Part model, mm, in its own coordinate system. Give positions to 0.01 mm unless a question says otherwise; leave off trailing zeros. Order: outer loops, then holes, each group sorted by start corner. A loop starts at its lowest first (then second) coordinate and runs counter-clockwise, first axis right, second up. Notation, with made-up numbers: M -16,68.5 L 19,68.5 A19 cw 19,99.5 Z; hole C -22,74.5 d8. An arc over 180 degrees is marked long. One line per question, with ' | ' between items.
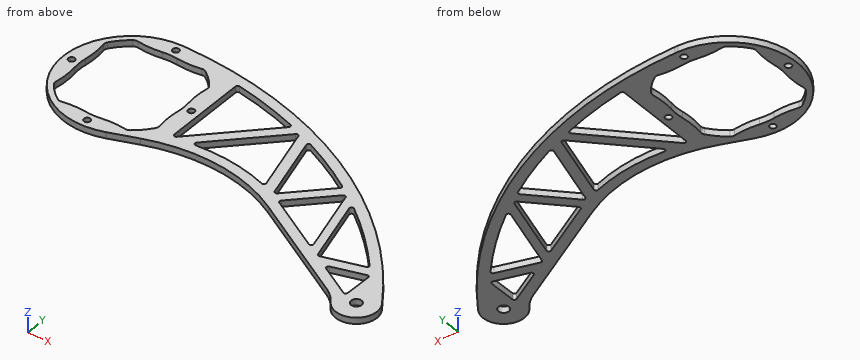
```python
from build123d import *

# Parameters (mm, degrees)
SKETCH_2_R          = 1.55
EXTRUDE_1_DEPTH     = 3
SKETCH_7_R          = 2.55
CUT_EXTRUDE_2_DEPTH = 5
CUT_EXTRUDE_4_DEPTH = 184.170177924
CUT_EXTRUDE_5_DEPTH = 184.170177924


with BuildPart() as part:
    # 草图2 → 凸台-拉伸1 (new body)
    with BuildSketch(Plane.XY):
        with BuildLine():
            Line((10.730362356, -31.206719208), (23.987000349, -26.648453139))
            ThreePointArc((23.987000349, -26.648453139), (58.3964084, -22.742948884), (91.232460283, -33.745404185))
            Line((91.232460283, -33.745404185), (142.367635598, -64.500382059))
            ThreePointArc((142.367635598, -64.500382059), (145.885654628, -67.188078585), (148.726187194, -70.583891486))
            ThreePointArc((148.726187194, -70.583891486), (162.505343691, -73.443257489), (165.49953058, -59.692767585))
            ThreePointArc((165.49953058, -59.692767585), (95.05641772, 7.182197604), (1.414573065, 32.983322541))
            ThreePointArc((1.414573065, 32.983322541), (0.707335687, 32.99583049), (0, 33))
            ThreePointArc((0, 33), (-32.548592395, -5.439589421), (10.730362356, -31.206719208))
        make_face()
        with Locations((-29, 0)):
            Circle(SKETCH_2_R, mode=Mode.SUBTRACT)
        with Locations((0, 29)):
            Circle(SKETCH_2_R, mode=Mode.SUBTRACT)
        with Locations((0, -29)):
            Circle(SKETCH_2_R, mode=Mode.SUBTRACT)
        with Locations((29, 0)):
            Circle(SKETCH_2_R, mode=Mode.SUBTRACT)
        with BuildLine():
            ThreePointArc((-17.479158967, 24.504877103), (-21.283914114, 21.283914114), (-24.504877103, 17.479158967))
            ThreePointArc((-24.504877103, 17.479158967), (-24.920981627, 16.556612715), (-24.953330783, 15.545085111))
            ThreePointArc((-24.953330783, 15.545085111), (-24.421536801, 9.520350069), (-24.806472783, 3.484452336))
            ThreePointArc((-24.806472783, 3.484452336), (-25.05, 0), (-24.806472783, -3.484452336))
            ThreePointArc((-24.806472783, -3.484452336), (-24.421536801, -9.520350069), (-24.953330783, -15.545085111))
            ThreePointArc((-24.953330783, -15.545085111), (-24.920981627, -16.556612715), (-24.504877103, -17.479158967))
            ThreePointArc((-24.504877103, -17.479158967), (-21.283914114, -21.283914114), (-17.479158967, -24.504877103))
            ThreePointArc((-17.479158967, -24.504877103), (-16.556612715, -24.920981627), (-15.545085111, -24.953330783))
            ThreePointArc((-15.545085111, -24.953330783), (-9.520350069, -24.421536801), (-3.484452336, -24.806472783))
            ThreePointArc((-3.484452336, -24.806472783), (0, -25.05), (3.484452336, -24.806472783))
            ThreePointArc((3.484452336, -24.806472783), (9.520350069, -24.421536801), (15.545085111, -24.953330783))
            ThreePointArc((15.545085111, -24.953330783), (16.556612715, -24.920981627), (17.479158967, -24.504877103))
            ThreePointArc((17.479158967, -24.504877103), (21.283914114, -21.283914114), (24.504877103, -17.479158967))
            ThreePointArc((24.504877103, -17.479158967), (24.920981627, -16.556612715), (24.953330783, -15.545085111))
            ThreePointArc((24.953330783, -15.545085111), (24.421536801, -9.520350069), (24.806472783, -3.484452336))
            ThreePointArc((24.806472783, -3.484452336), (25.05, 0), (24.806472783, 3.484452336))
            ThreePointArc((24.806472783, 3.484452336), (24.421536801, 9.520350069), (24.953330783, 15.545085111))
            ThreePointArc((24.953330783, 15.545085111), (24.920981627, 16.556612715), (24.504877103, 17.479158967))
            ThreePointArc((24.504877103, 17.479158967), (21.283914114, 21.283914114), (17.479158967, 24.504877103))
            ThreePointArc((17.479158967, 24.504877103), (16.556612715, 24.920981627), (15.545085111, 24.953330783))
            ThreePointArc((15.545085111, 24.953330783), (9.520350069, 24.421536801), (3.484452336, 24.806472783))
            ThreePointArc((3.484452336, 24.806472783), (0, 25.05), (-3.484452336, 24.806472783))
            ThreePointArc((-3.484452336, 24.806472783), (-9.520350069, 24.421536801), (-15.545085111, 24.953330783))
            ThreePointArc((-15.545085111, 24.953330783), (-16.556612715, 24.920981627), (-17.479158967, 24.504877103))
        make_face(mode=Mode.SUBTRACT)
    extrude(amount=EXTRUDE_1_DEPTH)

    # 草图7 → 切除-拉伸2 (cut)
    with BuildSketch(Plane.XY.offset(3)):
        with Locations((157.059520527, -65.056183502)):
            Circle(SKETCH_7_R)
    extrude(amount=-CUT_EXTRUDE_2_DEPTH, mode=Mode.SUBTRACT)

    # 草图9 → 切除-拉伸4 (cut, through all)
    with BuildSketch(Plane.XY.offset(3)):
        with BuildLine():
            Line((33, 23.419217625), (33, -16.604240946))
            ThreePointArc((33, -16.604240946), (33.617316568, -17.528120479), (34.707106781, -17.311347728))
            Line((34.707106781, -17.311347728), (65.868650079, 13.85019557))
            ThreePointArc((65.868650079, 13.85019557), (66.139078304, 14.768075481), (65.514441307, 15.492964147))
            ThreePointArc((65.514441307, 15.492964147), (50.039622799, 20.601738513), (34.192271497, 24.400559396))
            ThreePointArc((34.192271497, 24.400559396), (33.364496852, 24.191315902), (33, 23.419217625))
        make_face()
        with BuildLine():
            Line((70.777272632, 11.687750311), (43.285444418, -15.804077902))
            ThreePointArc((43.285444418, -15.804077902), (43.082610213, -16.925922432), (44.062405255, -17.508741905))
            ThreePointArc((44.062405255, -17.508741905), (62.271705947, -18.191622153), (79.917026283, -22.739987506))
            ThreePointArc((79.917026283, -22.739987506), (80.940663068, -22.54482321), (81.234917124, -21.545155305))
            Line((81.234917124, -21.545155305), (72.450305239, 11.239462575))
            ThreePointArc((72.450305239, 11.239462575), (71.743198458, 11.946569356), (70.777272632, 11.687750311))
        make_face()
        with BuildLine():
            Line((78.420751264, 8.275971191), (87.070117002, -24.003901194))
            ThreePointArc((87.070117002, -24.003901194), (87.777223783, -24.711007975), (88.743149609, -24.45218893))
            Line((88.743149609, -24.45218893), (106.170669274, -7.024669265))
            ThreePointArc((106.170669274, -7.024669265), (106.459042033, -6.222586245), (106.024202869, -5.489503085))
            ThreePointArc((106.024202869, -5.489503085), (93.207654626, 2.482542409), (79.812900532, 9.439408155))
            ThreePointArc((79.812900532, 9.439408155), (78.745415788, 9.302112816), (78.420751264, 8.275971191))
        make_face()
        with BuildLine():
            Line((109.945638003, -10.320768348), (92.838490747, -27.427915604))
            ThreePointArc((92.838490747, -27.427915604), (92.553025259, -28.256678823), (93.030191775, -28.991968654))
            Line((93.030191775, -28.991968654), (118.888407737, -44.544254432))
            ThreePointArc((118.888407737, -44.544254432), (120.005457191, -44.486072744), (120.369739316, -43.428489117))
            Line((120.369739316, -43.428489117), (111.61867061, -10.769056085))
            ThreePointArc((111.61867061, -10.769056085), (110.911563829, -10.061949303), (109.945638003, -10.320768348))
        make_face()
        with BuildLine():
            Line((117.134569213, -15.899856701), (125.688599687, -47.823933039))
            ThreePointArc((125.688599687, -47.823933039), (126.154525513, -48.431139397), (126.913344559, -48.53103982))
            Line((126.913344559, -48.53103982), (145.779824835, -43.475781666))
            ThreePointArc((145.779824835, -43.475781666), (146.474470094, -42.811361762), (146.288127832, -41.868354653))
            ThreePointArc((146.288127832, -41.868354653), (133.176898235, -27.681248062), (118.726274243, -14.861037407))
            ThreePointArc((118.726274243, -14.861037407), (117.553950154, -14.803607846), (117.134569213, -15.899856701))
        make_face()
        with BuildLine():
            Line((149.412514403, -47.678786332), (134.175652373, -51.761491208))
            ThreePointArc((134.175652373, -51.761491208), (133.444233225, -52.588031523), (133.919065665, -53.584363304))
            Line((133.919065665, -53.584363304), (148.921539819, -62.607521196))
            ThreePointArc((148.921539819, -62.607521196), (149.921379935, -62.625402537), (150.436785689, -61.768456267))
            Line((150.436785689, -61.768456267), (150.671173564, -48.662593499))
            ThreePointArc((150.671173564, -48.662593499), (150.287163938, -47.856833482), (149.412514403, -47.678786332))
        make_face()
    extrude(amount=-CUT_EXTRUDE_4_DEPTH, mode=Mode.SUBTRACT)

    # 草图10 → 切除-拉伸5 (cut, through all)
    with BuildSketch(Plane.XY.offset(3)):
        with BuildLine():
            ThreePointArc((-3.498362326, -24.905500618), (-9.519132496, -24.521529388), (-15.52876795, -25.051990553))
            ThreePointArc((-15.52876795, -25.051990553), (-16.579200462, -25.018397199), (-17.537229262, -24.586288654))
            ThreePointArc((-17.537229262, -24.586288654), (-21.354624792, -21.354624792), (-24.586288654, -17.537229262))
            ThreePointArc((-24.586288654, -17.537229262), (-25.018397199, -16.579200462), (-25.051990553, -15.52876795))
            ThreePointArc((-25.051990553, -15.52876795), (-24.521529388, -9.519132496), (-24.905500618, -3.498362326))
            ThreePointArc((-24.905500618, -3.498362326), (-25.15, 0), (-24.905500618, 3.498362326))
            ThreePointArc((-24.905500618, 3.498362326), (-24.521529388, 9.519132496), (-25.051990553, 15.52876795))
            ThreePointArc((-25.051990553, 15.52876795), (-25.018397199, 16.579200462), (-24.586288654, 17.537229262))
            ThreePointArc((-24.586288654, 17.537229262), (-21.354624792, 21.354624792), (-17.537229262, 24.586288654))
            ThreePointArc((-17.537229262, 24.586288654), (-16.579200462, 25.018397199), (-15.52876795, 25.051990553))
            ThreePointArc((-15.52876795, 25.051990553), (-9.519132496, 24.521529388), (-3.498362326, 24.905500618))
            ThreePointArc((-3.498362326, 24.905500618), (0, 25.15), (3.498362326, 24.905500618))
            ThreePointArc((3.498362326, 24.905500618), (9.519132496, 24.521529388), (15.52876795, 25.051990553))
            ThreePointArc((15.52876795, 25.051990553), (16.579200462, 25.018397199), (17.537229262, 24.586288654))
            ThreePointArc((17.537229262, 24.586288654), (21.354624792, 21.354624792), (24.586288654, 17.537229262))
            ThreePointArc((24.586288654, 17.537229262), (25.018397199, 16.579200462), (25.051990553, 15.52876795))
            ThreePointArc((25.051990553, 15.52876795), (24.521529388, 9.519132496), (24.905500618, 3.498362326))
            ThreePointArc((24.905500618, 3.498362326), (25.15, 0), (24.905500618, -3.498362326))
            ThreePointArc((24.905500618, -3.498362326), (24.521529388, -9.519132496), (25.051990553, -15.52876795))
            ThreePointArc((25.051990553, -15.52876795), (25.018397199, -16.579200462), (24.586288654, -17.537229262))
            ThreePointArc((24.586288654, -17.537229262), (21.354624792, -21.354624792), (17.537229262, -24.586288654))
            ThreePointArc((17.537229262, -24.586288654), (16.579200462, -25.018397199), (15.52876795, -25.051990553))
            ThreePointArc((15.52876795, -25.051990553), (9.519132496, -24.521529388), (3.498362326, -24.905500618))
            ThreePointArc((3.498362326, -24.905500618), (0, -25.15), (-3.498362326, -24.905500618))
        make_face()
    extrude(amount=-CUT_EXTRUDE_5_DEPTH, mode=Mode.SUBTRACT)


solid = part.part
```
1. Slice it at C-C on z = 2.45. Give the number of separate pieces and of enclosed holes in the cut face, then the cut area to 3 significant figures.
Worked out:
separate pieces: 1 | enclosed holes: 12 | area: 3,880 mm2
2. Slice it at B-B on y = -38. Give the cut face in (x, z), then the cut area to 3 significant figures.
Worked out:
outline: M 98.31,0 L 108.01,0 L 108.01,3 L 98.31,3 Z; M 118.92,0 L 123.06,0 L 123.06,3 L 118.92,3 Z; M 142.97,0 L 149.57,0 L 149.57,3 L 142.97,3 Z | area: 61.3 mm2
3. Drop flat-ended pins along their axis: pin 1 (3 mm diameter, centred on x = -29, y = 0, fed in from +Z) (3 decimals); pin 2 (1.5 mm diameter, centred on x = 27.5, z = 2.5, fed in from +Y); pin 3 (1 mm diameter, centred on x = 113, z = 1.5, fed in from -Y); pin 4 (1.5 mm diameter, centred on y = -36, z = 1.5, fed in from +X). Give the stop position or say it passes through.
Worked out:
pin 1: passes through | pin 2: stops at y = 30.77 | pin 3: stops at y = -47.14 | pin 4: stops at x = 148.51
4. Slice it at A-A on x = 140.5. Give the cut face in (y, z).
Worked out:
outline: M -63.38,0 L -57.54,0 L -57.54,3 L -63.38,3 Z; M -50.07,0 L -44.89,0 L -44.89,3 L -50.07,3 Z; M -35.26,0 L -27.96,0 L -27.96,3 L -35.26,3 Z
5. Probe L1, parallel to Y at x = 47.5, z = 1.75; L2, parallel to X at y = 4, z = 1.4; L3, parallel to Y at x = 140, z = 1.9. List the from-to ranges inside material, lowest first. Write a range as from..to.
Worked out:
L1: y = -22.34..-17.34, -11.59..-4.52, 21.31..26.48 | L2: x = -32.76..-24.84, 24.84..33, 56.02..63.09, 74.39..79.57, 90.49..100.49 | L3: y = -63.08..-57.24, -50.2..-45.02, -34.71..-27.44
